Part print with two shaded views. Sizes in mm from the minimum x, y, z corner. Round coordinates to 2 decimals unless told otherwise and drop trailing zeros. Order: outer loops, then holes, each group sorted by start corner. A loop starts at its lowest first (then second) coordinate and runs counter-clockwise, first axis right, second up. Notation, with made-up numbers: M 34,-14 L 90,-14 A21 cw 90,17 Z; hole C 48.25,3.5 d7. An arc over 180 degrees is marked long. One line per question, with ' | ' between items.
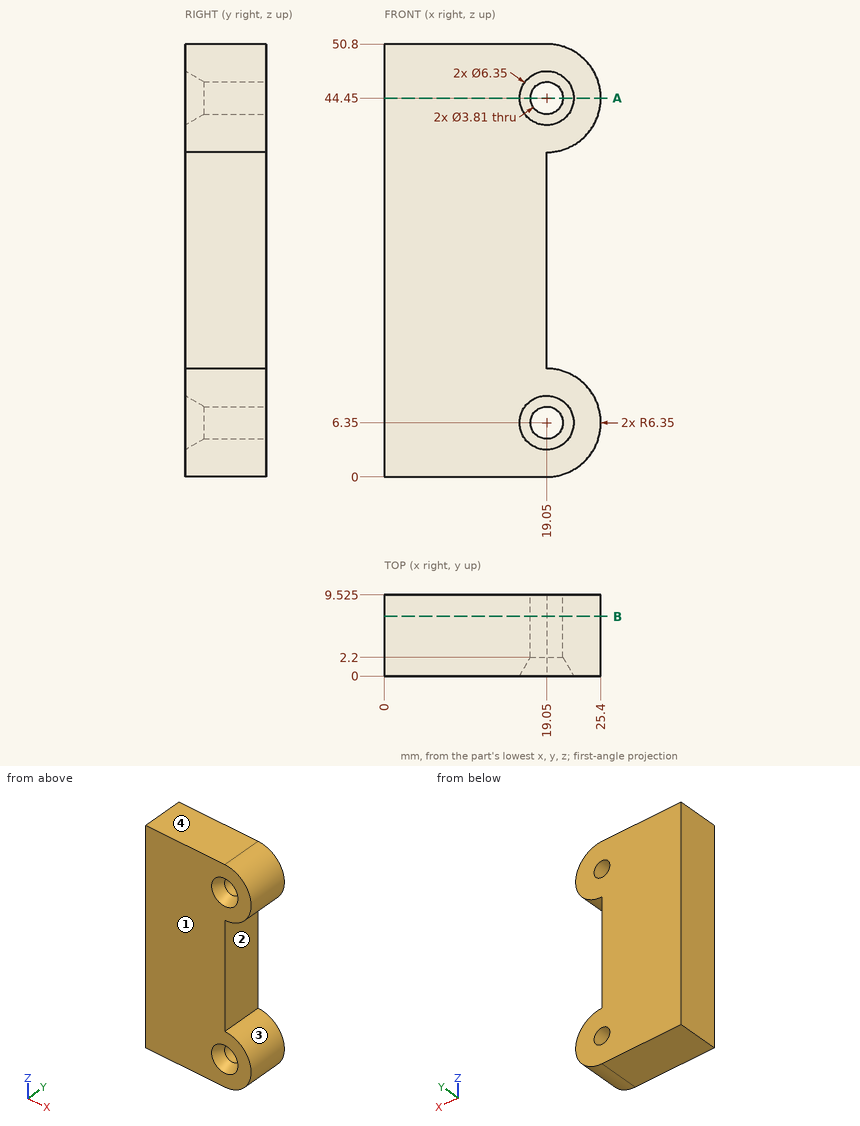
1) Saw through at B-B (y = 7). Give the number of separate pieces and of enclosed holes in the cut face, plus the area to 3 significant figures.
The answers:
separate pieces: 1 | enclosed holes: 2 | area: 1,070 mm²
2) Saw through at A-A (z = 44.45). List the corners of the cut face in (x, y) (1 decimal), plus the area to 3 significant figures.
The answers:
outline: M 0,0 L 15.9,0 L 17.1,2.2 L 17.1,9.5 L 0,9.5 Z; M 21,2.2 L 22.2,0 L 25.4,0 L 25.4,9.5 L 21,9.5 Z | area: 203 mm²
3) Two-plate mould, pull along Z, no slides. Class the marked faces 1, 2, 3 and 4: released by +Z, released by -Z, zero draft, split by the parting line, or undercut.
The answers:
face 1: zero draft | face 2: undercut | face 3: undercut | face 4: released by +Z
4) Probe line 1 (Z direction, x = 19.25, y = 5) (1 decimal); line 2 (X direction, y = 3.5, z = 6.35) (1 decimal); line 3 (X direction, y = 6.5, z = 29). List the from-to ranges inside material, lowest first. Write a range as [from, to].
The answers:
line 1: z = [0, 4.5], [8.2, 12.7], [38.1, 42.6], [46.3, 50.8] | line 2: x = [0, 17.1], [21, 25.4] | line 3: x = [0, 19.05]
5) Drop flat-ended pins along their axis: pin 1 (1 mm diameter, centred on y = 1, z = 42.5, fed in from +X); pin 2 (3 mm diameter, centred on y = 5.5, z = 21, fed in from +X); pin 3 (4.5 mm diameter, centred on x = 19.05, z = 6.35, fed in from -Y). Give the stop position or say it passes through.
The answers:
pin 1: stops at x = 25.23 | pin 2: stops at x = 19.05 | pin 3: stops at y = 1.6
